Autodesk Inventor part; units mm, degrees
ref_plane "YZ Plane" through (0, 0, 0) normal (1, 0, 0) x (0, 1, 0)
ref_plane "XZ Plane" through (0, 0, 0) normal (0, 1, 0) x (-1, 0, 0)
ref_plane "XY Plane" through (0, 0, 0) normal (0, 0, 1) x (1, 0, 0)
sketch "Sketch1" plane through (0, 0, 0) normal (0, 1, 0) x (-1, 0, 0)
  line L0 (0, -7) -> (-9, -7)
  line L1 (-18, -7) -> (-18, 0)
  line L2 (-18, 0) -> (-9, 0)
  line L3 (0, 0) -> (0, -7)
  line L4 (-9, -7) -> (-9, -2) construction
  line L5 (-9, -2) -> (-9, 0) construction
  circle A0 centre (-16, -2) radius 1
  line L6 (-16, -2) -> (-9, -2) construction
  line L7 (-9, 0) -> (0, 0)
  line L8 (-9, -7) -> (-18, -7)
  circle A1 centre (-2, -2) radius 1
  circle A2 centre (-35, -20) radius 1
  line L9 (-33, -15) -> (-51, -15)
  line L10 (-51, -15) -> (-51, -22)
  line L11 (-51, -22) -> (-33, -22)
  line L12 (-33, -22) -> (-33, -15)
  line L13 (-35, -20) -> (-35, -22) construction
  line L14 (-42, -15) -> (-42, -22) construction
  circle A3 centre (-49, -20) radius 1
  line L15 (-42, -15) -> (-9, -15)
  line L16 (-9, -15) -> (-9, -7)
  line L17 (-9, -7) -> (-42, -7)
  line L18 (-42, -7) -> (-42, -15)
  line L19 (-33, -15) -> (-16, -15)
  line L20 (-16, -15) -> (-16, -22)
  line L21 (-16, -22) -> (-33, -22)
  line L22 (-33, -22) -> (-33, -15)
  line L23 (-33, -7) -> (-18, -7)
  line L24 (-18, -7) -> (-18, 0)
  line L25 (-18, 0) -> (-33, 0)
  line L26 (-33, 0) -> (-33, -7)
  point P0 (0, 0)
  dimension "d0" = 18
  dimension "d1" = 7
  dimension "d2" = 2
  dimension "d4" = 7
  dimension "d11" = 0
  dimension "d12" = 2
  dimension "d17" = 0
  dimension "d18" = 2
  dimension "d19" = 19
  dimension "d20" = 18
  dimension "d21" = 7
  dimension "d22" = 2
  dimension "d23" = 7
  dimension "d24" = 18
  dimension "d27" = 16
  dimension "d28" = 22
extrude "Extrusion2" add sketch "Sketch1" along normal blind 3
properties part number "game-switch-holder"
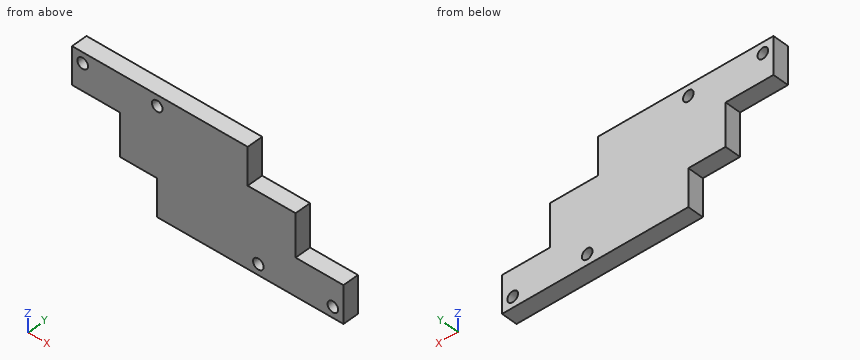
The listing builds one solid part. Answer for the finished solid, in the listing's coordinates (mm). Round coordinates to 2 decimals unless told otherwise and drop trailing zeros. Order: outer loops, then holes, each group sorted by start corner. A loop starts at its lowest first (then second) coordinate and runs counter-clockwise, first axis right, second up. Notation, with made-up numbers: (43.25, 61) -> (50.25, 61) arc R22 ccw to (50.25, 92) -> close; hole circle Ø6 at (25.5, 5.5). An arc over 180 degrees is marked (long way). Answer as CSV lines item,"result". Start each with the question number.
(1) The part is cut by section B-B (x = 35). Determine the outline of the cut face in (y, z), then the cut area to 3 significant figures.
(2) The part is cut by section D-D (x = 49). Determine the outline of the cut face in (y, z).
(3) Find the intervals of material crossed by probe 1 along Z at (x, y) = (35, 1.8); probe 2 along X at (y, z) = (1.1, -20.5); probe 3 along Z at (x, y) = (38, 0.7), in increasing order. Write a range as from..to.
(4) The part is cut by section A-A (z = -20). Determine the outline of the cut face in (x, y), then the cut area to 3 significant figures.
(5) The part is cut by section C-C (y = 2.05). Determine the outline of the cut face in (x, z), then the cut area to 3 significant figures.
(6) Flat-ended cylindrical pins translate along their axes: pin 1 Ø1 at (y, z) = (2.5, -11) entering from -X; pin 2 Ø0.9 at (x, y) = (5, 1) entering from -Z; pin 3 Ø1 at (y, z) = (0.5, -3) entering from +X. Find the tip coordinate at first contact, or state that the pin passes through.
Evaluation:
1,outline,"(0, -22) -> (3, -22) -> (3, -21) -> (0, -21) -> close; (0, -19) -> (3, -19) -> (3, -7) -> (0, -7) -> close"
1,area,"39.0 mm²"
2,outline,"(0, -22) -> (3, -22) -> (3, -21) -> (0, -21) -> close; (0, -19) -> (3, -19) -> (3, -15) -> (0, -15) -> close"
3,probe 1,"-22..-21, -19..-7"
3,probe 2,"16..34.13, 35.87..48.13, 49.87..51"
3,probe 3,"-22..-7"
4,outline,"(16, 0) -> (34, 0) -> (34, 3) -> (16, 3) -> close; (36, 0) -> (48, 0) -> (48, 3) -> (36, 3) -> close; (50, 0) -> (51, 0) -> (51, 3) -> (50, 3) -> close"
4,area,"93.0 mm²"
5,outline,"(0, -7) -> (9, -7) -> (9, -15) -> (16, -15) -> (16, -22) -> (51, -22) -> (51, -15) -> (42, -15) -> (42, -7) -> (33, -7) -> (33, 0) -> (0, 0) -> close; hole circle Ø2 at (2, -2); hole circle Ø2 at (16, -2); hole circle Ø2 at (35, -20); hole circle Ø2 at (49, -20)"
5,area,"727 mm²"
6,pin 1,"x = 9"
6,pin 2,"z = -7"
6,pin 3,"x = 33"
